Source: CAD feature listing. Evaluate the final solid. Frame: model axes, mm. A direction names the side the tool comes from. Coordinates: 2 decimals unless noted, no trailing zeros. Loops run counter-clockwise (first coordinate to the right, second up) from the corner with the lowest first, then second, coordinate; pieces in that order, holes last.
Item 1: Reachability of faces 4 (the cylindrical face through (6.05, -5.5, 1.86)), 5 (the flat face through (8.8, 0, -1)), 6 (the flat face through (1, 6.05, -1)) from +Z, -Z, +X, -X, +Y, -Y: full face, straight path, thin tool, end or side. Return the list, or none.
Item 2: Pin query (flat end, axial travel): pin 1 Ø9 at (x, y) = (-3, -1.5) entering from -Z; pin 2 Ø0.6 at (x, z) = (5.5, 0) entering from -Y; pin 3 Ø0.8 at (x, z) = (-1, -1) entering from +Y; pin 4 Ø0.6 at (x, y) = (5.5, -8.5) entering from -Z. Return the tip coordinate at first contact, or that it passes through.
Item 3: Section query A-A, the plane y = 0.8. State how many separate pieces and enclosed holes the cut face has, then the cut area to 3 significant figures.
Item 4: Section query B-B, the plane x = 5.5. Return the cut outline in (y, z).
Item 5: Line query: probe 1 along X at (y, z) = (-1, -0.9); probe 2 along Y at (x, z) = (0.75, -0.15); probe 3 along X at (y, z) = (6.25, -1.05). Output: solid intervals per line, ascending.
Item 6: Pull-direction query (Y, two-part tool) for faces 1 (the flat face through (0, -9.05, 2)), 2 (the flat face through (1, 0, 3.67)), 3 (the cylindrical face through (-4.05, -1.18, 1.86)); classes: +Y half, -Y half, draft (parallel to the pull), parting line (faces both ways), or undercut.
```python
from build123d import *

# Parameters (mm, degrees)
BOSS_EXTRUDE1_DEPTH = 3.67
SKETCH6_R           = 0.5
CUT_EXTRUDE1_DEPTH  = 3.67
SKETCH20_W          = 12.1
SKETCH20_H          = 12.1
BOSS_EXTRUDE4_DEPTH = 1.5
SKETCH13_W          = 1
SKETCH13_H          = 0.5
CUT_EXTRUDE7_DEPTH  = 0.5
SKETCH14_R          = 0.125
CUT_EXTRUDE8_DEPTH  = 0.25
CUT_EXTRUDE9_START  = -0.25
SKETCH15_R          = 0.125
CUT_EXTRUDE9_DEPTH  = 0.25
CUT_EXTRUDE10_START = -0.25
SKETCH16_R          = 0.125
CUT_EXTRUDE10_DEPTH = 0.25
SKETCH17_R          = 0.125
CUT_EXTRUDE11_DEPTH = 0.25
SKETCH19_W          = 3.67
SKETCH19_H          = 18.1
CUT_EXTRUDE13_DEPTH = 0.125
CUT_EXTRUDE14_REACH = 22.457


with BuildPart() as part:
    # Sketch1 → Boss-Extrude1 (new body)
    with BuildSketch(Plane.XY):
        with BuildLine():
            Line((-7.8, 9.05), (7.8, 9.05))
            ThreePointArc((7.8, 9.05), (9.567766953, 8.317766953), (10.3, 6.55))
            Line((10.3, 6.55), (10.3, -6.55))
            ThreePointArc((10.3, -6.55), (9.567766953, -8.317766953), (7.8, -9.05))
            Line((7.8, -9.05), (-7.8, -9.05))
            Line((-7.8, -9.05), (-7.8, 9.05))
        make_face()
    extrude(amount=BOSS_EXTRUDE1_DEPTH)

    # Sketch6 → Cut-Extrude1 (cut)
    with BuildSketch(Plane.XY.offset(3.67)):
        with Locations((-3.55, 4.8)):
            Circle(SKETCH6_R)
        with Locations((-1.55, 4.8)):
            Circle(SKETCH6_R)
        with Locations((0.45, 4.8)):
            Circle(SKETCH6_R)
        with Locations((2.45, 4.8)):
            Circle(SKETCH6_R)
        with Locations((4.45, 4.8)):
            Circle(SKETCH6_R)
        with Locations((6.45, 4.8)):
            Circle(SKETCH6_R)
        with Locations((-1.55, 2.8)):
            Circle(SKETCH6_R)
        with Locations((0.45, 2.8)):
            Circle(SKETCH6_R)
        with Locations((2.45, 2.8)):
            Circle(SKETCH6_R)
        with Locations((4.45, 2.8)):
            Circle(SKETCH6_R)
        with Locations((6.45, 2.8)):
            Circle(SKETCH6_R)
        with Locations((-1.55, 0.8)):
            Circle(SKETCH6_R)
        with Locations((0.45, 0.8)):
            Circle(SKETCH6_R)
        with Locations((2.45, 0.8)):
            Circle(SKETCH6_R)
        with Locations((4.45, 0.8)):
            Circle(SKETCH6_R)
        with Locations((6.45, 0.8)):
            Circle(SKETCH6_R)
        with Locations((-1.55, -1.2)):
            Circle(SKETCH6_R)
        with Locations((0.45, -1.2)):
            Circle(SKETCH6_R)
        with Locations((2.45, -1.2)):
            Circle(SKETCH6_R)
        with Locations((4.45, -1.2)):
            Circle(SKETCH6_R)
        with Locations((6.45, -1.2)):
            Circle(SKETCH6_R)
        with Locations((-1.55, -3.2)):
            Circle(SKETCH6_R)
        with Locations((0.45, -3.2)):
            Circle(SKETCH6_R)
        with Locations((2.45, -3.2)):
            Circle(SKETCH6_R)
        with Locations((4.45, -3.2)):
            Circle(SKETCH6_R)
        with Locations((6.45, -3.2)):
            Circle(SKETCH6_R)
        with Locations((-1.55, -5.2)):
            Circle(SKETCH6_R)
        with Locations((0.45, -5.2)):
            Circle(SKETCH6_R)
        with Locations((2.45, -5.2)):
            Circle(SKETCH6_R)
        with Locations((4.45, -5.2)):
            Circle(SKETCH6_R)
        with Locations((6.45, -5.2)):
            Circle(SKETCH6_R)
        with Locations((-3.55, 2.8)):
            Circle(SKETCH6_R)
        with Locations((-3.55, 0.8)):
            Circle(SKETCH6_R)
        with Locations((-3.55, -1.2)):
            Circle(SKETCH6_R)
        with Locations((-3.55, -3.2)):
            Circle(SKETCH6_R)
        with Locations((-3.55, -5.2)):
            Circle(SKETCH6_R)
    extrude(amount=-CUT_EXTRUDE1_DEPTH, mode=Mode.SUBTRACT)

    # Sketch20 → Boss-Extrude4 (add)
    with BuildSketch(Plane(origin=(0, 0, 0), x_dir=(-1, 0, 0), z_dir=(0, 0, -1))):
        with BuildLine():
            Line((6.3, -7.55), (6.3, 7.55))
            Line((6.3, 7.55), (-7.8, 7.55))
            ThreePointArc((-7.8, 7.55), (-8.507106781, 7.257106781), (-8.8, 6.55))
            Line((-8.8, 6.55), (-8.8, -6.55))
            ThreePointArc((-8.8, -6.55), (-8.507106781, -7.257106781), (-7.8, -7.55))
            Line((-7.8, -7.55), (6.3, -7.55))
        make_face()
        with Locations((-1.25, 0)):
            Rectangle(SKETCH20_W, SKETCH20_H, mode=Mode.SUBTRACT)
    extrude(amount=BOSS_EXTRUDE4_DEPTH)

    # Sketch13 → Cut-Extrude7 (cut)
    with BuildSketch(Plane.XZ.offset(9.05)):
        with Locations((-5.5, 0.25)):
            Rectangle(SKETCH13_W, SKETCH13_H)
        with Locations((5.5, 0.25)):
            Rectangle(SKETCH13_W, SKETCH13_H)
    extrude(amount=-CUT_EXTRUDE7_DEPTH, mode=Mode.SUBTRACT)

    # Sketch14 → Cut-Extrude8 (cut)
    with BuildSketch(Plane(origin=(-6, 0, 0), x_dir=(0, 0, -1), z_dir=(1, 0, 0))):
        with Locations(Location((-0.25, -8.8, 0), (0, 0, 90))):
            Circle(SKETCH14_R)
    extrude(amount=-CUT_EXTRUDE8_DEPTH, mode=Mode.SUBTRACT)

    # Sketch15 → Cut-Extrude9 (cut)
    with BuildSketch(Plane.ZY.offset(5).offset(CUT_EXTRUDE9_START)):
        with Locations(Location((0.25, -8.8, 0), (0, 0, 90))):
            Circle(SKETCH15_R)
    extrude(amount=CUT_EXTRUDE9_DEPTH, mode=Mode.SUBTRACT)

    # Sketch16 → Cut-Extrude10 (cut)
    with BuildSketch(Plane.ZY.offset(-6).offset(CUT_EXTRUDE10_START)):
        with Locations(Location((0.25, -8.8, 0), (0, 0, 90))):
            Circle(SKETCH16_R)
    extrude(amount=CUT_EXTRUDE10_DEPTH, mode=Mode.SUBTRACT)

    # Sketch17 → Cut-Extrude11 (cut)
    with BuildSketch(Plane(origin=(5, 0, 0), x_dir=(0, 0, -1), z_dir=(1, 0, 0))):
        with Locations(Location((-0.25, -8.8, 0), (0, 0, 90))):
            Circle(SKETCH17_R)
    extrude(amount=-CUT_EXTRUDE11_DEPTH, mode=Mode.SUBTRACT)

    # Sketch19 → Cut-Extrude13 (cut)
    with BuildSketch(Plane.ZY.offset(7.8)):
        with Locations((1.835, 0)):
            Rectangle(SKETCH19_W, SKETCH19_H)
    extrude(amount=-CUT_EXTRUDE13_DEPTH, mode=Mode.SUBTRACT)

    # Sketch21 → Cut-Extrude14 (cut, up to next)
    with BuildSketch(Plane.ZY.offset(7.675), mode=Mode.PRIVATE) as cut_extrude14_sk1:
        with BuildLine():
            Line((0, -8.55), (0, -9.05))
            Line((0, -9.05), (0.5, -9.05))
            ThreePointArc((0.5, -9.05), (0.146446609, -8.903553391), (0, -8.55))
        make_face()
    cut_extrude14_tool1 = extrude(cut_extrude14_sk1.sketch, amount=-CUT_EXTRUDE14_REACH, mode=Mode.PRIVATE) & part.part
    add(cut_extrude14_tool1.solids().sort_by_distance((-7.675, -8.938316, 0.111684))[0], mode=Mode.SUBTRACT)
    add(cut_extrude14_tool1.solids().sort_by_distance((-7.675, -8.938316, 0.111684))[1], mode=Mode.SUBTRACT)
    add(cut_extrude14_tool1.solids().sort_by_distance((-7.675, -8.938316, 0.111684))[2], mode=Mode.SUBTRACT)


solid = part.part
```
Verdict:
1. face 4: +Z, -Z
1. face 5: -Z, +X, +Y, -Y
1. face 6: -Z
2. pin 1: stops at z = -1.5
2. pin 2: stops at y = -8.55
2. pin 3: stops at y = 7.55
2. pin 4: stops at z = 0
3. separate pieces: 7
3. enclosed holes: 0
3. area: 48.4 mm2
4. outline: (-9.05, 0.5) - (-8.55, 0.5) - (-8.55, 0) - (-7.55, 0) - (-7.55, -1.5) - (-6.05, -1.5) - (-6.05, 0) - (6.05, 0) - (6.05, -1.5) - (7.55, -1.5) - (7.55, 0) - (9.05, 0) - (9.05, 3.67) - (-9.05, 3.67) - close
5. probe 1: x = -6.3 to -4.8, 7.3 to 8.8
5. probe 2: y = -7.55 to -6.05, 6.05 to 7.55
5. probe 3: x = -6.3 to 8.8
6. face 1: -Y half
6. face 2: draft
6. face 3: undercut
